```python
from build123d import *

# Parameters (mm, degrees)
SKETCH1_W           = 40
SKETCH1_H           = 6.35
BOSS_EXTRUDE1_DEPTH = 6.35
SKETCH2_R           = 3.2
CUT_EXTRUDE1_DEPTH  = 6.35


with BuildPart() as part:
    # Sketch1 → Boss-Extrude1 (new body)
    with BuildSketch(Plane(origin=(0, 0, 0), x_dir=(1, 0, 0), z_dir=(0, 1, 0))):
        with BuildLine():
            Line((171.132486541, 50), (128.867513459, 123.205080757))
            ThreePointArc((128.867513459, 123.205080757), (92.264973081, 159.807621135), (42.264973081, 173.205080757))
            Line((42.264973081, 173.205080757), (-42.264973081, 173.205080757))
            ThreePointArc((-42.264973081, 173.205080757), (-92.264973081, 159.807621135), (-128.867513459, 123.205080757))
            Line((-128.867513459, 123.205080757), (-171.132486541, 50))
            ThreePointArc((-171.132486541, 50), (-184.529946162, 0), (-171.132486541, -50))
            Line((-171.132486541, -50), (-128.867513459, -123.205080757))
            ThreePointArc((-128.867513459, -123.205080757), (-92.264973081, -159.807621135), (-42.264973081, -173.205080757))
            Line((-42.264973081, -173.205080757), (42.264973081, -173.205080757))
            ThreePointArc((42.264973081, -173.205080757), (92.264973081, -159.807621135), (128.867513459, -123.205080757))
            Line((128.867513459, -123.205080757), (171.132486541, -50))
            ThreePointArc((171.132486541, -50), (184.529946162, 0), (171.132486541, 50))
        make_face()
        with Locations((0, -153.175)):
            Rectangle(SKETCH1_W, SKETCH1_H, mode=Mode.SUBTRACT)
        Polygon((-139.903810568, -57.679491924), (-145.403071882, -60.854491924), (-125.403071882, -95.495508076), (-119.903810568, -92.320508076), align=None, mode=Mode.SUBTRACT)
        Polygon((-119.903810568, 92.320508076), (-125.403071882, 95.495508076), (-145.403071882, 60.854491924), (-139.903810568, 57.679491924), align=None, mode=Mode.SUBTRACT)
        with Locations((0, 153.175)):
            Rectangle(SKETCH1_W, SKETCH1_H, mode=Mode.SUBTRACT)
        Polygon((139.903810568, 57.679491924), (145.403071882, 60.854491924), (125.403071882, 95.495508076), (119.903810568, 92.320508076), align=None, mode=Mode.SUBTRACT)
        Polygon((119.903810568, -92.320508076), (125.403071882, -95.495508076), (145.403071882, -60.854491924), (139.903810568, -57.679491924), align=None, mode=Mode.SUBTRACT)
    extrude(amount=BOSS_EXTRUDE1_DEPTH)

    # Sketch2 → Cut-Extrude1 (cut)
    with BuildSketch(Plane(origin=(0, 6.35, 0), x_dir=(1, 0, 0), z_dir=(0, 1, 0))):
        with Locations(Location((55.794244464, -33.346698257, 0), (0, 0, 270))):
            Circle(SKETCH2_R)
        with Locations(Location((-56.776210055, -31.645883963, 0), (0, 0, 270))):
            Circle(SKETCH2_R)
        with Locations(Location((0.981965591, 64.99258222, 0), (0, 0, 270))):
            Circle(SKETCH2_R)
    extrude(amount=-CUT_EXTRUDE1_DEPTH, mode=Mode.SUBTRACT)


solid = part.part
```
The listing builds one solid part. Answer for the finished solid, in the listing's coordinates (mm). A direction names the side the tool comes from. Coordinates: 2 decimals unless noted, no trailing zeros. Loops run counter-clockwise (first coordinate to the right, second up) from the corner with the lowest first, then second, coordinate; pieces in that order, holes last. Notation, with made-up numbers: (79, 55.5) - (99, 55.5) arc R22 ccw to (99, 65.5) - close; hole circle Ø6 at (-17.5, 69.25). An arc over 180 degrees is marked (long way). Use a Markdown table: item, result. Add a question column.
1) The part is cut by section D-D, the plane z = 129. Give the vertices of the cut face in (x, y), and give its area (3 significant figures).
2) Find the intervals of material crossed by line 1 (Z direction, x = 9, y = 2.5); line 2 (Z direction, x = 129, y = 1); line 3 (X direction, y = 3.5, z = 86), in increasing order.
3) The mould has two halves that part along X. Classify faces 3 (the flat face through (135.26, 3.13, 78.42)), 4 (the cylindrical face through (-91.63, 3.13, -160.17)), 5 (the cylindrical face through (92.9, 3.13, -159.44)), 6 (the flat face through (-135.543, 3.131, 77.933)): released by +X, released by -X, zero draft, split by the parting line, or undercut.
4) The part is cut by section C-C, the plane y = 2.5. State how many separate pieces and enclosed holes the cut face has, and give its area (3 significant figures).
5) Given pin 1 (1 mm diameter, centred on y = 5, z = -2, fed in from -X); pin 2 (1.9 mm diameter, centred on y = 4.5, z = -151.5, fed in from -X); pin 3 (4 mm diameter, centred on x = 55.79, z = 33.35, fed in from +Y); pin 4 (2 mm diameter, centred on y = 3, z = -55.5, fed in from -X), each flat-ended and moving along its own axis, determine where each tip first touches the part or whether it passes through.
6) The part is cut by section B-B, the plane x = -156. Give the vertices of the cut face in (y, z), and give its area (3 significant figures).
7) For faces 1 (the flat face through (130.044, 3.131, 74.758)), 2 (the cylindrical face through (184.527, 3.131, 0.733)), determine the directions among +Z, -Z, +X, -X, +Y, -Y from which every point of the face is accessible in a straight line to the end or side of a thin tool.
8) The part is cut by section A-A, the plane z = 83. Give the vertices of the cut face in (x, y) (3 decimals).
Here are the results:
| question | item | result |
|---|---|---|
| 1 | outline | (-125.25, 0) - (125.25, 0) - (125.25, 6.35) - (-125.25, 6.35) - close |
| 1 | area | 1,590 mm^2 |
| 2 | line 1 | z = -173.21 to -156.35, -150 to 150, 156.35 to 173.21 |
| 2 | line 2 | z = -122.98 to -89.27, -76.57 to 76.57, 89.27 to 122.98 |
| 2 | line 3 | x = -150.35 to -130.89, -123.55 to 123.55, 130.89 to 150.35 |
| 3 | face 3 | undercut |
| 3 | face 4 | released by -X |
| 3 | face 5 | released by +X |
| 3 | face 6 | undercut |
| 4 | separate pieces | 1 |
| 4 | enclosed holes | 9 |
| 4 | area | 99,100 mm^2 |
| 5 | pin 1 | stops at x = -184.52 |
| 5 | pin 2 | stops at x = -105.65 |
| 5 | pin 3 | passes through |
| 5 | pin 4 | stops at x = -168.53 |
| 6 | outline | (0, -76.21) - (6.35, -76.21) - (6.35, 76.21) - (0, 76.21) - close |
| 6 | area | 968 mm^2 |
| 7 | face 1 | +Y, -Y |
| 7 | face 2 | +X, +Y, -Y |
| 8 | outline | (-152.08, 0) - (-132.617, 0) - (-132.617, 6.35) - (-152.08, 6.35) - close; (-125.285, 0) - (125.285, 0) - (125.285, 6.35) - (-125.285, 6.35) - close; (132.617, 0) - (152.08, 0) - (152.08, 6.35) - (132.617, 6.35) - close |
